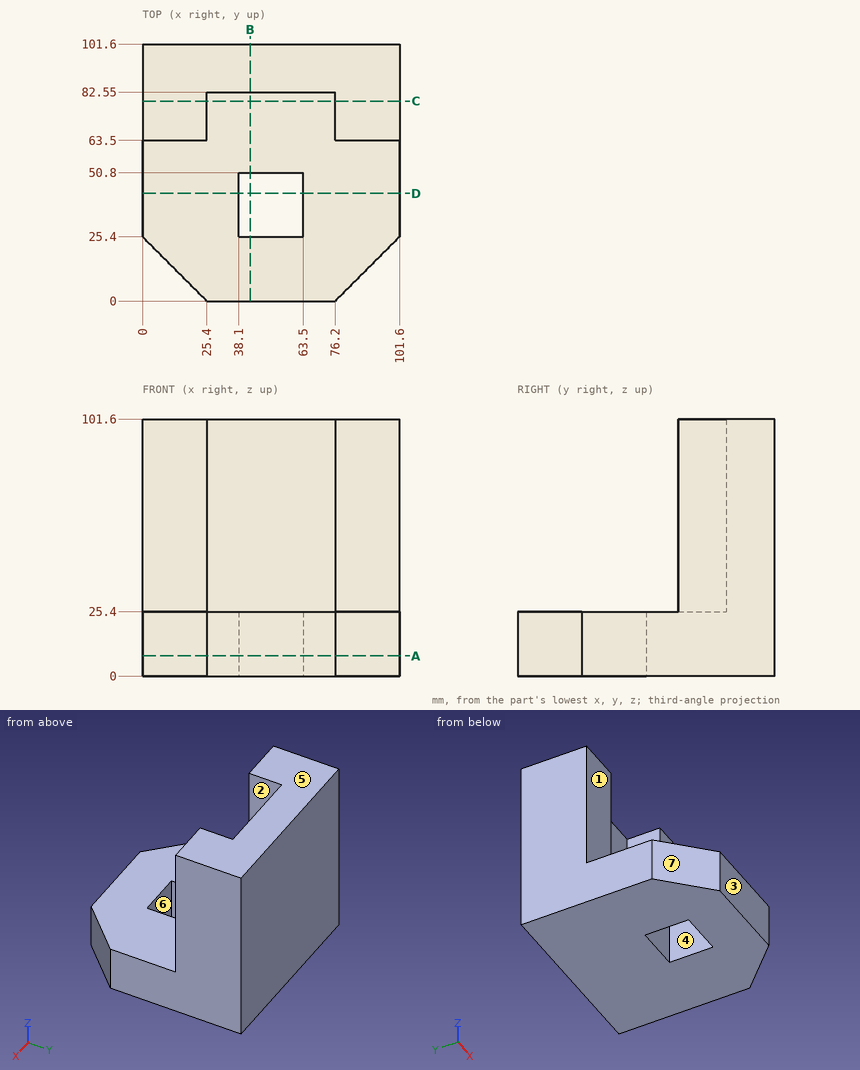
Study the drawing (mm; zero at the part's minimum x, y, z) and answer. A direction names the side the tool comes from. Give positions to 0.01 mm unless a question says otherwise; leave off trailing zeros. Order: outer loops, then holes, each group sorted by start corner. A loop starts at its lowest first (then second) coordinate and runs counter-clockwise, first axis right, second up. Notation, with made-up numbers: M -19,75.5 L 10,75.5 A20 ccw 10,82.5 Z; hole C -6,-0.75 d4. An arc over 180 degrees is marked long. Put each result on its own line as item: value. Start each with the question number.
Item 1: The part is cut by section A-A, the plane z = 8. Determine the outline of the cut face in (x, y).
Item 2: The part is cut by section D-D, the plane y = 42.5. Determine the outline of the cut face in (x, z), and give its area (3 significant figures).
Item 3: Find the intervals of material crossed by line 1 along Y through (x, z) = (55, 22); line 2 along X through (y, z) = (78.5, 97.5); line 3 along Y through (x, z) = (5, 75), in increasing order.
Item 4: The part is cut by section B-B, the plane x = 42.5. Determine the outline of the cut face in (y, z).
Item 5: Which of the six approach directions +Z, -Z, +X, -X, +Y, -Y give full straight-line access (tool end or side, diameter ignored) to the marked faces 1, 2, 3 and 4?
Item 6: The part is cut by section C-C, the plane y = 79. Determine the outline of the cut face in (x, z).
Item 7: For a pull along X with two mould halves and no side action, classify the marked faces 5, 6 and 7 as +X half, -X half, draft (parallel to the pull), parting line (faces both ways), or undercut.
Item 8: Flat-ended cylindrical pins translate along their axes: P1, Ø15, axis at x = 57.5, z = 44.5, coming from the -Y side; P2, Ø5, axis at x = 13, y = 42.5, coming from the +Z side; P3, Ø12.5, axis at x = 91, z = 45.5, coming from the -Y side. Find the tip coordinate at first contact, or state that the pin passes through.
Answer key:
1. outline: M 0,25.4 L 25.4,0 L 76.2,0 L 101.6,25.4 L 101.6,101.6 L 0,101.6 Z; hole M 38.1,25.4 L 63.5,25.4 L 63.5,50.8 L 38.1,50.8 Z
2. outline: M 0,0 L 38.1,0 L 38.1,25.4 L 0,25.4 Z; M 63.5,0 L 101.6,0 L 101.6,25.4 L 63.5,25.4 Z
2. area: 1,940 mm²
3. line 1: y = 0 to 25.4, 50.8 to 101.6
3. line 2: x = 0 to 25.4, 76.2 to 101.6
3. line 3: y = 63.5 to 101.6
4. outline: M 0,0 L 25.4,0 L 25.4,25.4 L 0,25.4 Z; M 50.8,0 L 101.6,0 L 101.6,101.6 L 82.55,101.6 L 82.55,25.4 L 50.8,25.4 Z
5. face 1: +Z, +X, -X, -Y
5. face 2: +Z, -Y
5. face 3: +Z, -Z, +X, -X, -Y
5. face 4: +Z, -Z
6. outline: M 0,0 L 101.6,0 L 101.6,101.6 L 76.2,101.6 L 76.2,25.4 L 25.4,25.4 L 25.4,101.6 L 0,101.6 Z
7. face 5: draft
7. face 6: undercut
7. face 7: -X half
8. P1: stops at y = 82.55
8. P2: stops at z = 25.4
8. P3: stops at y = 63.5
